Drawing for the job (mm, zero at the part's lowest x, y, z). Coordinates: 2 decimals unless noted, no trailing zeros. Order: outer loops, then holes, each group sorted by start corner. A loop starts at its lowest first (then second) coordinate and runs counter-clockwise, first axis right, second up. Notation, with made-up numbers: (15.5, -30.75) -> (34.5, -30.75) arc R20 cw to (34.5, -14.75) -> close; hole circle Ø2 at (-27.75, 22). An arc over 180 degrees is marked (long way). Write each question's results on one line, items separated by ' | '.
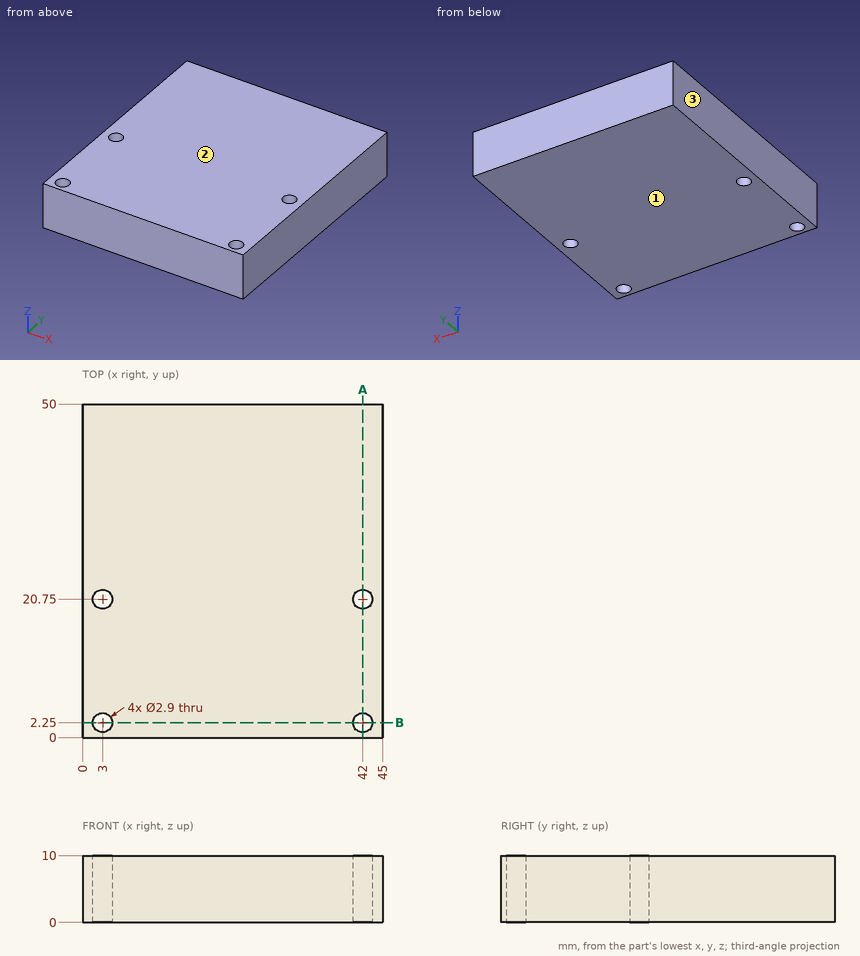
Item 1: Pull direction Z, two halves, no side cores. Call the marked faces 1, 2 and 3: released by +Z, released by -Z, zero draft, split by the parting line, or undercut.
Answer:
face 1: released by -Z | face 2: released by +Z | face 3: zero draft
Item 2: Drill centre lines: line 1 (Y direction, x = 3, z = 5); line 2 (X direction, y = 3, z = 2.5); line 3 (Y direction, x = 43, z = 7.25). Where is each one in solid material? Low to high. Write a range as from..to.
Answer:
line 1: y = 0..0.8, 3.7..19.3, 22.2..50 | line 2: x = 0..1.76, 4.24..40.76, 43.24..45 | line 3: y = 0..1.2, 3.3..19.7, 21.8..50
Item 3: Slice it at A-A, the plane x = 42. List the corners of the cut face in (y, z), and give its area (3 significant figures).
Answer:
outline: (0, 0) -> (0.8, 0) -> (0.8, 10) -> (0, 10) -> close; (3.7, 0) -> (19.3, 0) -> (19.3, 10) -> (3.7, 10) -> close; (22.2, 0) -> (50, 0) -> (50, 10) -> (22.2, 10) -> close | area: 442 mm^2
Item 4: Pin check, flat tip, straight feed: pin 1 (2.5 mm diameter, centred on x = 3, y = 20.75, fed in from +Z). Stop position of the tip, or through.
Answer:
pin 1: passes through
Item 5: Slice it at B-B, the plane y = 2.25. List the corners of the cut face in (x, z).
Answer:
outline: (0, 0) -> (1.55, 0) -> (1.55, 10) -> (0, 10) -> close; (4.45, 0) -> (40.55, 0) -> (40.55, 10) -> (4.45, 10) -> close; (43.45, 0) -> (45, 0) -> (45, 10) -> (43.45, 10) -> close
